For this review, take the finished solid that the model builds, in its own axes (mm). A direction names the side the tool comes from. Give positions to 0.01 mm unless a question says otherwise; leave off trailing zeros. Write each loop counter-clockwise with the first axis right and the second up, starting at its lowest first coordinate (ties: lowest second). Pieces come first, ordered by that corner, then holes.
1) Machinability: for faces 1 (the face through (0, -12, 1.588)), 2 (the face through (-1.588, -12, 2)), 3 (the face through (1.588, -13, 2)), which of the approach directions +Z, -Z, +X, -X, +Y, -Y give a long, thin tool a straight path to every point of the face, cutting with its end or side? Answer none if there is none.
2) Wall thickness on line 1 along Z through (x, y) = (0, -12.6); line 2 along Y through (x, z) = (1.3, 2.9); line 3 along Y through (x, z) = (-1.75, 0.8): over which ranges is each line inside the solid? List them lowest first.
3) We need section D-D on z = 0.5. Give the boundary of the cut face in (x, y), and give its area (3 significant figures).
4) We need section B-B on y = -1.5. Give the boundary of the cut face in (x, z) (1 decimal).
5) We need section C-C on x = 2. Give the boundary of the cut face in (y, z) (1 decimal).
6) Draft analysis for pull direction Y (two halves, no side actions). For faces 4 (the face through (0, -1, 3.175)), 5 (the face through (0, -13.295, 4)), 6 (the face through (0, 13, 0)), state which applies: pulls with the +Y half, pulls with the -Y half, needs draft (parallel to the pull), parting line crosses it, or undercut.
7) For P1, Ø2.5, axis at x = 0, y = 3.5, coming from the -Z side (3 decimals); P2, Ø0.8, axis at x = 0.5, y = -13, coming from the -Z side, all flat-tipped, find the tip position at first contact; note any pin that passes through.
from build123d import *

# Parameters (mm, degrees)
F0_W     = 4.7625
F0_H     = 26.590625
F1_DEPTH = 4.7625
F3_DEPTH = 3.175
F4_DEPTH = 1.5875
F5_R     = 0.396875
F6_DEPTH = 1.5885


with BuildPart() as f1:
    # F0 (on Top) → F1 (new body)
    with BuildSketch(Plane.XY):
        Rectangle(F0_W, F0_H)
    extrude(amount=F1_DEPTH)

    # F2 (on face) → F3 (cut)
    with BuildSketch(Plane(origin=(0, 0, 0), x_dir=(1, 0, 0), z_dir=(0, 0, -1))):
        Polygon((-2.38125, -11.7078125), (2.38125, -11.7078125), (2.38125, 13.2953125), (1.5875, 13.2953125), (1.5875, 11.7078125), (-1.5875, 11.7078125), (-1.5875, 13.2953125), (-2.38125, 13.2953125), align=None)
    extrude(amount=-F3_DEPTH, mode=Mode.SUBTRACT)

    # F4 (cut): a face of the model
    f4_faces = [f1.faces().sort_by_distance(p)[0] for p in [
        (0, -12.5015625, 0),
    ]]
    extrude(f4_faces, amount=-F4_DEPTH, mode=Mode.SUBTRACT)

    # F5 (on face) → F6 (cut, through all)
    with BuildSketch(Plane(origin=(0, -11.7078125, 0), x_dir=(-1, 0, 0), z_dir=(0, 1, 0))):
        with Locations((0, 2.38125)):
            Circle(F5_R)
    extrude(amount=-F6_DEPTH, mode=Mode.SUBTRACT)


solid = f1.part
Results list:
1. face 1: -Z, +X, -X, -Y
1. face 2: -Z, -X, -Y
1. face 3: -Z, +X, -Y
2. line 1: z = 1.59 to 1.98, 2.78 to 4.76
2. line 2: y = -13.3 to -11.71, 11.71 to 13.3
2. line 3: y = 11.71 to 13.3
3. outline: (-2.38, 11.71) - (2.38, 11.71) - (2.38, 13.3) - (-2.38, 13.3) - close
3. area: 7.56 mm2
4. outline: (-2.4, 3.2) - (2.4, 3.2) - (2.4, 4.8) - (-2.4, 4.8) - close
5. outline: (-13.3, 3.2) - (11.7, 3.2) - (11.7, 0) - (13.3, 0) - (13.3, 4.8) - (-13.3, 4.8) - close
6. face 4: undercut
6. face 5: pulls with the -Y half
6. face 6: needs draft
7. P1: stops at z = 3.175
7. P2: stops at z = 1.59
